Geometry: final body of the model. Coordinates: model frame, mm. Round coordinates to 2 decimals unless told otherwise and drop trailing zeros. Write each loop counter-clockwise with the first axis right and the second up, starting at its lowest first coordinate (ties: lowest second). Pieces come first, ordered by that corner, then holes.
Autodesk Inventor part; units mm, degrees
ref_plane "YZ Plane" through (0, 0, 0) normal (1, 0, 0) x (0, 1, 0)
ref_plane "XZ Plane" through (0, 0, 0) normal (0, 1, 0) x (-1, 0, 0)
ref_plane "XY Plane" through (0, 0, 0) normal (0, 0, 1) x (1, 0, 0)
sketch "Sketch1" plane through (0, 0, 0) normal (0, 0, 1) x (1, 0, 0)
  line L0 (203.2, -76.2) -> (-203.2, -76.2)
  line L1 (-203.2, -76.2) -> (-203.2, 76.2)
  line L2 (-203.2, 76.2) -> (203.2, 76.2)
  line L3 (203.2, 76.2) -> (203.2, -76.2)
  line L4 (203.2, -76.2) -> (-203.2, 76.2) construction
  line L5 (-203.2, -76.2) -> (203.2, 76.2) construction
  line L6 (149.225, -76.2) -> (174.625, -76.2)
  line L7 (174.625, -76.2) -> (174.625, -114.3)
  line L8 (174.625, -114.3) -> (149.225, -114.3)
  line L9 (149.225, -114.3) -> (149.225, -76.2)
  line L10 (0, 0) -> (203.2, 0) construction
  line L11 (174.625, 76.2) -> (174.625, 114.3)
  line L12 (174.625, 114.3) -> (149.225, 114.3)
  line L13 (149.225, 114.3) -> (149.225, 76.2)
  line L14 (-203.2, -76.2) -> (-177.8, -76.2)
  line L15 (-177.8, -76.2) -> (-177.8, -114.3)
  line L16 (-177.8, -114.3) -> (-203.2, -114.3)
  line L17 (-203.2, -114.3) -> (-203.2, -76.2)
  line L18 (149.225, -114.3) -> (149.225, -76.2)
  line L19 (-177.8, 76.2) -> (-177.8, 114.3)
  line L20 (-177.8, 114.3) -> (-203.2, 114.3)
  line L21 (-203.2, 114.3) -> (-203.2, 76.2)
  dimension "d0" = 406.4
  dimension "d1" = 152.4
  dimension "d2" = 25.4
  dimension "d3" = 38.1
  dimension "d4" = 28.575
  dimension "d6" = 25.4
  dimension "d7" = 38.1
extrude "Plate1" add sketch "Sketch1" along normal blind 3.048
sketch "Sketch2" plane through (0, 0, 3.048) normal (0, 0, 1) x (1, 0, 0)
  line L0 (-203.2, -114.3) -> (-203.2, 114.3) construction
  line L1 (-177.8, -114.3) -> (-203.2, -114.3) construction
  line L2 (-177.8, -76.2) -> (-177.8, -114.3) construction
  line L3 (149.225, -76.2) -> (-177.8, -76.2) construction
  line L4 (149.225, -114.3) -> (149.225, -76.2) construction
  line L5 (174.625, -114.3) -> (149.225, -114.3) construction
  line L6 (174.625, -76.2) -> (174.625, -114.3) construction
  line L7 (203.2, -76.2) -> (174.625, -76.2) construction
  line L8 (203.2, 76.2) -> (203.2, -76.2) construction
  line L9 (174.625, 76.2) -> (203.2, 76.2) construction
  line L10 (174.625, 114.3) -> (174.625, 76.2) construction
  line L11 (149.225, 114.3) -> (174.625, 114.3) construction
  line L12 (149.225, 76.2) -> (149.225, 114.3) construction
  line L13 (-177.8, 76.2) -> (149.225, 76.2) construction
  line L14 (-177.8, 114.3) -> (-177.8, 76.2) construction
  line L15 (-203.2, 114.3) -> (-177.8, 114.3) construction
  point P0 (0, 0)
  point P1 (-190.5, 101.6)
  point P2 (161.925, 101.6)
  point P3 (-190.5, -101.6)
  point P4 (161.925, -101.6)
  dimension "d8" = 12.7
  dimension "d9" = 12.7
  dimension "d12" = 352.425
  dimension "d15" = 203.2
hole "Hole1" at (-190.5, 101.6, 3.048) at (161.925, 101.6, 3.048) at (-190.5, -101.6, 3.048) at (161.925, -101.6, 3.048) direction (0, 0, -1) diameter 5.1054 end through all
equation "\"d23\" = Thickness"
equation "\"d5\" = Thickness"
equation "\"BendRadius\" = Thickness"
equation "\"BendReliefWidth\" = Thickness"
equation "\"BendReliefDepth\" = 0.5 * Thickness"
equation "\"CornerReliefSize\" = 4 * Thickness"
equation "\"MinimumRemnant\" = 2 * Thickness"
equation "\"TransitionRadius\" = BendRadius"
equation "\"JacobiRadiusSize\" = BendRadius"
equation "\"GapSize\" = Thickness"
properties part number "feeder_slide_plate" material "Polycarbonate, Clear"
1) First-contact query: P1, Ø1.5, axis at x = 7.5, z = 1, coming from the +Y side; P2, Ø4.5, axis at x = 161.925, y = -101.6, coming from the -Z side; P3, Ø0.9, axis at y = -90.5, z = 1, coming from the +X side (3 decimals); P4, Ø1, axis at x = -137, z = 2.5, coming from the -Y side. Flat tips, straight axial feed; report the tip coordinate or a pass-through.
2) Section A-A on x = 130.5. Output: boundary loops of the cut face in (y, z), plus the area to 3 significant figures.
3) Line query: probe 1 along X at (y, z) = (-101.6, 1.35) (3 decimals); probe 2 along X at (y, z) = (-102, 0.9) (3 decimals); probe 3 along Y at (x, z) = (-190.5, 2). Output: solid intervals per line, ascending.
Filled in:
1. P1: stops at y = 76.2
1. P2: passes through
1. P3: stops at x = 174.625
1. P4: stops at y = -76.2
2. outline: (-76.2, 0) - (76.2, 0) - (76.2, 3.05) - (-76.2, 3.05) - close
2. area: 465 mm2
3. probe 1: x = -203.2 to -193.053, -187.947 to -177.8, 149.225 to 159.372, 164.478 to 174.625
3. probe 2: x = -203.2 to -193.021, -187.979 to -177.8, 149.225 to 159.404, 164.446 to 174.625
3. probe 3: y = -114.3 to -104.15, -99.05 to 99.05, 104.15 to 114.3
